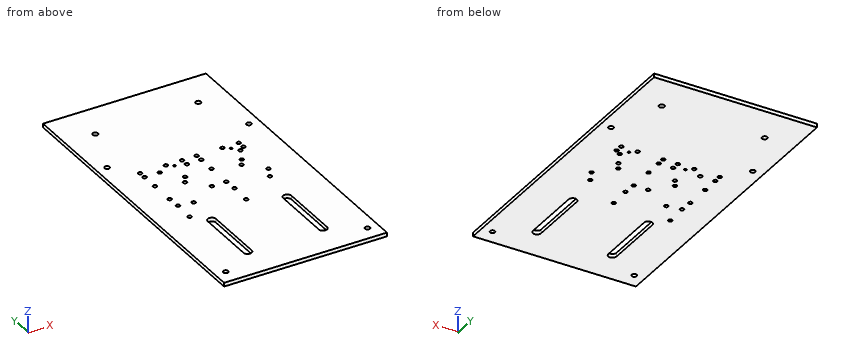
Autodesk Inventor part; units mm, degrees
ref_plane "YZ Plane" through (0, 0, 0) normal (1, 0, 0) x (0, 1, 0)
ref_plane "XZ Plane" through (0, 0, 0) normal (0, 1, 0) x (-1, 0, 0)
ref_plane "XY Plane" through (0, 0, 0) normal (0, 0, 1) x (1, 0, 0)
sketch "Sketch1" plane through (0, 0, 0) normal (0, 0, 1) x (1, 0, 0)
  line L0 (-68.58, -128.7145) -> (68.58, -128.7145)
  line L1 (68.58, -128.7145) -> (68.58, 128.7145)
  line L2 (68.58, 128.7145) -> (-68.58, 128.7145)
  line L3 (-68.58, 128.7145) -> (-68.58, -128.7145)
  line L4 (-68.58, -128.7145) -> (68.58, 128.7145) construction
  line L5 (68.58, -128.7145) -> (-68.58, 128.7145) construction
  point P0 (0, 0)
  dimension "d0" = 137.16
  dimension "d1" = 257.429
extrude "Extrusion1" add sketch "Sketch1" against normal blind 3.175
sketch "Sketch2" plane through (0, 0, 0) normal (0, 0, 1) x (1, 0, 0)
  circle A0 centre (-59.69, 52.5145) radius 2.0955
  line L0 (-68.58, 128.7145) -> (-68.58, -128.7145)
  line L1 (-68.58, 128.7145) -> (68.58, 128.7145)
  circle A1 centre (59.69, 52.5145) radius 2.0955
  line L2 (68.58, -128.7145) -> (68.58, 128.7145)
  circle A2 centre (-59.69, -116.0145) radius 2.0955
  circle A3 centre (59.69, -116.0145) radius 2.0955
  line L3 (-68.58, -128.7145) -> (68.58, -128.7145)
  point P0 (0, 0)
  dimension "d4" = 8.89
  dimension "d5" = 76.2
  dimension "d6" = 76.2
  dimension "d7" = 8.89
  dimension "d8" = 4.191
  dimension "d9" = 12.7
  dimension "d10" = 8.89
  dimension "d11" = 8.89
  dimension "d12" = 12.7
  dimension "d13" = 4.191
  dimension "d21" = 4.191
  dimension "d22" = 4.191
hole "Hole1" at (-59.69, 52.5145, 0) at (59.69, 52.5145, 0) at (-59.69, -116.0145, 0) at (59.69, -116.0145, 0) direction (0, 0, -1) diameter 4.191 end through all
sketch "Sketch4" plane through (0, 0, 0) normal (0, 0, 1) x (1, 0, 0)
  line L0 (-35.179, -49.0855) -> (-35.179, -99.8855)
  line L1 (-28.321, -49.0855) -> (-28.321, -99.8855)
  line L2 (28.321, -49.0855) -> (28.321, -99.8855)
  line L3 (35.179, -49.0855) -> (35.179, -99.8855)
  line L4 (-68.58, 128.7145) -> (-68.58, -128.7145)
  line L5 (68.58, -128.7145) -> (68.58, 128.7145)
  line L6 (-68.58, -128.7145) -> (68.58, -128.7145)
  arc A0 (-28.321, -49.0855) -> (-35.179, -49.0855) centre (-31.75, -49.0855) ccw
  arc A1 (-35.179, -99.8855) -> (-28.321, -99.8855) centre (-31.75, -99.8855) ccw
  arc A2 (35.179, -49.0855) -> (28.321, -49.0855) centre (31.75, -49.0855) ccw
  arc A3 (28.321, -99.8855) -> (35.179, -99.8855) centre (31.75, -99.8855) ccw
  point P0 (0, 0)
  dimension "d23" = 6.858
  dimension "d24" = 6.858
  dimension "d25" = 33.401
  dimension "d26" = 50.8
  dimension "d27" = 33.401
  dimension "d28" = 28.829
  dimension "d29" = 28.829
  dimension "d30" = 28.829
  dimension "d31" = 28.829
  dimension "d32" = 50.8
  dimension "d33" = 50.8
  dimension "d34" = 50.8
extrude "Extrusion2" cut sketch "Sketch4" against normal blind 3.175
sketch "Sketch5" plane through (0, 0, 0) normal (0, 0, 1) x (1, 0, 0)
  line L0 (-68.58, 128.7145) -> (68.58, 128.7145)
  line L1 (68.58, 128.7145) -> (68.58, -128.7145)
  point P0 (0, 0)
  point P1 (-43.3324, 96.9645)
  point P2 (43.3324, 96.9645)
  dimension "d37" = 31.75
  dimension "d38" = 86.6648
  dimension "d39" = 31.75
  dimension "d40" = 25.2476
hole "Hole2" at (-43.3324, 96.9645, 0) at (43.3324, 96.9645, 0) direction (0, 0, -1) diameter 4.4704 end through all
sketch "battery_buzzer" plane through (0, 0, 0) normal (0, 0, 1) x (1, 0, 0)
  line L0 (-50.8, 39.8145) -> (50.8, 39.8145)
  line L1 (50.8, 39.8145) -> (50.8, -36.3855)
  line L2 (50.8, -36.3855) -> (-50.8, -36.3855)
  line L3 (-50.8, -36.3855) -> (-50.8, 39.8145)
  line L4 (68.58, -128.7145) -> (68.58, 128.7145)
  line L5 (68.58, 128.7145) -> (-68.58, 128.7145)
  line L6 (-68.58, 128.7145) -> (-68.58, -128.7145)
  line L7 (-46.99, 37.2745) -> (-13.97, 37.2745)
  line L8 (-13.97, 37.2745) -> (-13.97, 9.3345)
  line L9 (-13.97, 9.3345) -> (-46.99, 9.3345)
  line L10 (-46.99, 9.3345) -> (-46.99, 37.2745)
  circle A0 centre (-43.18, 33.4645) radius 1.651
  circle A1 centre (-43.18, 12.5095) radius 1.651
  circle A2 centre (-17.78, 12.5095) radius 1.651
  line L11 (0.635, 37.2745) -> (33.655, 37.2745)
  line L12 (33.655, 37.2745) -> (33.655, 9.3345)
  line L13 (33.655, 9.3345) -> (0.635, 9.3345)
  line L14 (0.635, 9.3345) -> (0.635, 37.2745)
  circle A3 centre (4.445, 33.4645) radius 1.651
  circle A4 centre (4.445, 12.5095) radius 1.651
  circle A5 centre (29.845, 12.5095) radius 1.651
  point P0 (-1.6153, -4.4833)
  point P1 (48.3688, -4.4833)
  dimension "d48" = 17.78
  dimension "d49" = 88.9
  dimension "d50" = 76.2
  dimension "d51" = 17.78
  dimension "d52" = 33.02
  dimension "d54" = 3.302
  dimension "d55" = 3.302
  dimension "d57" = 3.81
  dimension "d58" = 3.81
  dimension "d59" = 3.81
  dimension "d60" = 20.955
  dimension "d62" = 25.4
  dimension "d74" = 33.02
  dimension "d75" = 3.302
  dimension "d76" = 3.302
  dimension "d77" = 3.81
  dimension "d78" = 3.81
  dimension "d79" = 3.81
  dimension "d80" = 20.955
  dimension "d81" = 25.4
  dimension "d190" = 25.4
  dimension "d191" = 95.25
  dimension "d192" = 73.025
sketch "grizzly_bear" plane through (0, 0, 0) normal (0, 0, 1) x (1, 0, 0)
  line L0 (-5.08, -39.9415) -> (-5.08, 36.2585)
  line L1 (-5.08, 36.2585) -> (-46.355, 36.2585)
  line L2 (-46.355, 36.2585) -> (-46.355, -39.9415)
  line L3 (-46.355, -39.9415) -> (-5.08, -39.9415)
  circle A0 centre (-43.18, -36.8935) radius 1.651
  circle A1 centre (-7.874, 33.4645) radius 1.651
  circle A2 centre (-43.18, 33.4645) radius 1.651
  line L4 (42.545, -39.9415) -> (42.545, 36.2585)
  line L5 (42.545, 36.2585) -> (1.27, 36.2585)
  line L6 (1.27, 36.2585) -> (1.27, -39.9415)
  line L7 (1.27, -39.9415) -> (42.545, -39.9415)
  circle A3 centre (4.445, -36.8935) radius 1.651
  circle A4 centre (39.751, 33.4645) radius 1.651
  circle A5 centre (4.445, 33.4645) radius 1.651
  line L8 (-68.58, 128.7145) -> (-68.58, -128.7145)
  line L9 (68.58, 128.7145) -> (-68.58, 128.7145)
  point P0 (0, 0)
  point P1 (53.9394, 0)
  dimension "d83" = 3.302
  dimension "d85" = 76.2
  dimension "d86" = 41.275
  dimension "d89" = 2.794
  dimension "d90" = 3.175
  dimension "d91" = 2.794
  dimension "d92" = 38.481
  dimension "d97" = 73.152
  dimension "d98" = 3.175
  dimension "d166" = 3.302
  dimension "d168" = 76.2
  dimension "d169" = 41.275
  dimension "d172" = 2.794
  dimension "d173" = 3.175
  dimension "d174" = 2.794
  dimension "d175" = 38.481
  dimension "d180" = 73.152
  dimension "d181" = 3.175
  dimension "d182" = 6.35
  dimension "d188" = 95.25
  dimension "d189" = 25.4
sketch "Smartsensor" plane through (0, 0, 0) normal (0, 0, 1) x (1, 0, 0)
  line L0 (-46.99, 9.3345) -> (-46.99, 37.2745)
  line L1 (-46.99, 37.2745) -> (-13.97, 37.2745)
  line L2 (-13.97, 37.2745) -> (-13.97, 9.3345)
  line L3 (-46.99, 9.3345) -> (-13.97, 9.3345)
  circle A0 centre (-43.18, 33.4645) radius 1.651
  circle A1 centre (-17.78, 12.5095) radius 1.651
  circle A2 centre (-16.51, 29.6545) radius 1
  line L4 (0.635, 9.3345) -> (0.635, 37.2745)
  line L5 (0.635, 37.2745) -> (33.655, 37.2745)
  line L6 (33.655, 37.2745) -> (33.655, 9.3345)
  line L7 (0.635, 9.3345) -> (33.655, 9.3345)
  circle A3 centre (4.445, 33.4645) radius 1.651
  circle A4 centre (29.845, 12.5095) radius 1.651
  circle A5 centre (31.115, 29.6545) radius 1
  point P0 (0, 0)
  point P1 (4.445, 33.4645)
sketch "SmartsensorPowered" plane through (0, 0, 0) normal (0, 0, 1) x (1, 0, 0)
  line L0 (-46.355, 36.6395) -> (-18.415, 36.6395)
  line L1 (-18.415, 36.6395) -> (-18.415, -23.0505)
  line L2 (-18.415, -23.0505) -> (-46.355, -23.0505)
  line L3 (-46.355, -23.0505) -> (-46.355, 36.6395)
  circle A0 centre (-43.18, 33.4645) radius 1.651
  circle A1 centre (-21.59, 33.4645) radius 1.651
  circle A2 centre (-42.545, -19.2405) radius 1.651
  circle A3 centre (-21.59, 6.1595) radius 1.651
  line L4 (-68.58, 128.7145) -> (-68.58, -128.7145)
  line L5 (68.58, 128.7145) -> (-68.58, 128.7145)
  line L6 (1.27, 36.6395) -> (29.21, 36.6395)
  line L7 (29.21, 36.6395) -> (29.21, -23.0505)
  line L8 (29.21, -23.0505) -> (1.27, -23.0505)
  line L9 (1.27, -23.0505) -> (1.27, 36.6395)
  circle A4 centre (4.445, 33.4645) radius 1.651
  circle A5 centre (26.035, 33.4645) radius 1.651
  circle A6 centre (5.08, -19.2405) radius 1.651
  circle A7 centre (26.035, 6.1595) radius 1.651
  dimension "d99" = 59.69
  dimension "d100" = 27.94
  dimension "d101" = 3.302
  dimension "d102" = 3.302
  dimension "d103" = 3.302
  dimension "d104" = 3.302
  dimension "d105" = 3.175
  dimension "d106" = 3.81
  dimension "d107" = 3.175
  dimension "d108" = 3.81
  dimension "d109" = 3.175
  dimension "d110" = 3.175
  dimension "d111" = 3.175
  dimension "d112" = 30.48
  dimension "d186" = 25.4
  dimension "d187" = 95.25
  dimension "d193" = 59.69
  dimension "d194" = 27.94
  dimension "d195" = 3.302
  dimension "d196" = 3.302
  dimension "d197" = 3.302
  dimension "d198" = 3.302
  dimension "d199" = 3.175
  dimension "d200" = 3.81
  dimension "d201" = 3.175
  dimension "d202" = 3.81
  dimension "d203" = 3.175
  dimension "d204" = 3.175
  dimension "d205" = 3.175
  dimension "d206" = 30.48
  dimension "d207" = 73.025
sketch "teamflag" plane through (0, 0, 0) normal (0, 0, 1) x (1, 0, 0)
  line L0 (-45.72, 29.6545) -> (-5.08, 29.6545)
  line L1 (-5.08, 29.6545) -> (-5.08, -10.9855)
  line L2 (-5.08, -10.9855) -> (-45.72, -10.9855)
  line L3 (-45.72, -10.9855) -> (-45.72, 29.6545)
  circle A0 centre (-43.18, 27.1145) radius 1.651
  circle A1 centre (-43.18, -8.4455) radius 1.651
  circle A2 centre (-7.62, 27.1145) radius 1.651
  circle A3 centre (-7.62, -8.4455) radius 1.651
  line L4 (1.905, 29.6545) -> (42.545, 29.6545)
  line L5 (42.545, 29.6545) -> (42.545, -10.9855)
  line L6 (42.545, -10.9855) -> (1.905, -10.9855)
  line L7 (1.905, -10.9855) -> (1.905, 29.6545)
  circle A4 centre (4.445, 27.1145) radius 1.651
  circle A5 centre (4.445, -8.4455) radius 1.651
  circle A6 centre (40.005, 27.1145) radius 1.651
  circle A7 centre (40.005, -8.4455) radius 1.651
  line L8 (-68.58, 128.7145) -> (-68.58, -128.7145)
  line L9 (68.58, 128.7145) -> (-68.58, 128.7145)
  point P0 (0, 0)
  point P1 (-43.18, 33.4645)
  point P2 (4.445, 33.4645)
  point P3 (-42.545, -19.2405)
  point P4 (5.08, -19.2405)
  point P5 (-43.18, 33.4645)
  point P6 (4.445, 27.1145)
  dimension "d128" = 40.64
  dimension "d129" = 40.64
  dimension "d140" = 35.56
  dimension "d141" = 35.56
  dimension "d142" = 35.56
  dimension "d143" = 2.54
  dimension "d144" = 2.54
  dimension "d145" = 40.64
  dimension "d146" = 40.64
  dimension "d147" = 35.56
  dimension "d148" = 35.56
  dimension "d149" = 35.56
  dimension "d150" = 2.54
  dimension "d151" = 2.54
  dimension "d209" = 25.4
  dimension "d210" = 101.6
  dimension "d211" = 73.025
  dimension "d212" = 101.6
sketch "cape" plane through (0, 0, 0) normal (0, 0, 1) x (1, 0, 0)
  line L0 (-33.655, 30.2793) -> (38.4048, 30.2793)
  line L1 (38.4048, 30.2793) -> (38.4048, -24.3205)
  line L2 (38.4048, -24.3205) -> (-33.655, -24.3205)
  line L3 (-33.655, -24.3205) -> (-33.655, 30.2793)
  circle A0 centre (-30.48, 27.1145) radius 1.5875
  circle A1 centre (-30.48, -21.1455) radius 1.5875
  circle A2 centre (35.56, 23.9395) radius 1.5875
  circle A3 centre (35.56, -17.9705) radius 1.5875
  line L4 (-68.58, 128.7145) -> (-68.58, -128.7145)
  point P0 (0, 0)
  point P1 (-43.18, 33.4645)
  point P2 (-43.18, 27.1145)
  point P3 (-42.545, -19.2405)
  point P4 (-30.48, 27.1145)
  point P5 (-24.13, 20.7645)
  dimension "d152" = 3.175
  dimension "d153" = 72.0598
  dimension "d154" = 54.5998
  dimension "d155" = 48.26
  dimension "d156" = 0
  dimension "d157" = 3.175
  dimension "d158" = 3.175
  dimension "d159" = 41.91
  dimension "d160" = 0
  dimension "d161" = 6.35
  dimension "d162" = 2.8448
  dimension "d269" = 38.1
  dimension "d270" = 44.45
sketch "Board Area" plane through (0, 0, 0) normal (0, 0, 1) x (1, 0, 0)
  line L0 (-50.8, 39.8145) -> (50.8, 39.8145)
  line L1 (50.8, 39.8145) -> (50.8, -128.7145)
  line L2 (50.8, -128.7145) -> (-50.8, -128.7145)
  line L3 (-50.8, -128.7145) -> (-50.8, 39.8145)
  line L4 (68.58, 128.7145) -> (-68.58, 128.7145)
  line L5 (-68.58, 128.7145) -> (-68.58, -128.7145)
  line L6 (-68.58, -128.7145) -> (68.58, -128.7145)
  point P0 (0, 0)
  dimension "d163" = 101.6
  dimension "d164" = 88.9
  dimension "d165" = 17.78
hole "Hole3" at (-43.18, 27.1145, 0) at (-43.18, -8.4455, 0) at (-7.62, -8.4455, 0) at (-7.62, 27.1145, 0) at (4.445, 27.1145, 0) at (4.445, -8.4455, 0) at (40.005, -8.4455, 0) at (40.005, 27.1145, 0) direction (0, 0, -1) diameter 3.302 end through all
hole "Hole5" at (-43.18, -36.8935, 0) at (4.445, -36.8935, 0) at (39.751, 33.4645, 0) at (-7.874, 33.4645, 0) direction (0, 0, -1) diameter 3.302 end through all
hole "Hole6" at (-17.78, 12.5095, 0) at (29.845, 12.5095, 0) direction (0, 0, -1) diameter 3.302 end through all
hole "Hole7" at (-43.18, 12.5095, 0) at (4.445, 12.5095, 0) direction (0, 0, -1) diameter 3.302 end through all
hole "Hole9" at (-43.18, 33.4645, 0) at (4.445, 33.4645, 0) at (-16.51, 29.6545, 0) direction (0, 0, -1) diameter 2.0066 end through all
hole "Hole10" at (31.115, 29.6545, 0) direction (0, 0, -1) diameter 2.0066 end through all
hole "Hole11" at (-30.48, 27.1145, 0) at (-30.48, -21.1455, 0) at (35.56, -17.9705, 0) at (35.56, 23.9395, 0) direction (0, 0, -1) diameter 3.302 end through all
hole "Hole12" at (-42.545, -19.2405, 0) at (-21.59, 33.4645, 0) at (26.035, 33.4645, 0) at (5.08, -19.2405, 0) at (4.445, 33.4645, 0) at (-43.18, 33.4645, 0) at (-21.59, 6.1595, 0) at (26.035, 6.1595, 0) direction (0, 0, -1) diameter 3.302 end through all
Geometry: final body of the model. Coordinates: model frame, mm. Coordinates: 2 decimals unless noted, no trailing zeros. Loops run counter-clockwise (first coordinate to the right, second up) from the corner with the lowest first, then second, coordinate; pieces in that order, holes last. Notation, with made-up numbers: M 27.25,71.25 L 60.25,71.25 A33 ccw 60.25,110.25 Z; hole C -32,-25 d6. An arc over 180 degrees is marked long. One line per item, written item: value. Start each with the question number.
1) Cut plane B-B (z = -2.25). Count the separate pieces of the cut face and the enclosed holes in it, then the cut area to 3 significant figures.
2) Cut plane A-A (y = -73). Return loops of the section in (x, z) (3 decimals).
3) Pin query (flat end, axial travel): P1, Ø2.5, axis at x = 4.44, y = 33.46, coming from the -Z side. Return the tip coordinate at first contact, or that it passes through.
4) Material intervals for L1, parallel to X at y = 6, z = -2.9; L2, parallel to X at y = -65.5, z = -0.4; L3, parallel to Y at x = -60, z = -3, sorted ascending. Write a range as from..to.
Evaluation:
1. separate pieces: 1
1. enclosed holes: 38
1. area: 34,200 mm^2
2. outline: M -68.58,-3.175 L -35.179,-3.175 L -35.179,0 L -68.58,0 Z; M -28.321,-3.175 L 28.321,-3.175 L 28.321,0 L -28.321,0 Z; M 35.179,-3.175 L 68.58,-3.175 L 68.58,0 L 35.179,0 Z
3. P1: through
4. L1: -68.58..-23.23, -19.95..24.39, 27.68..68.58
4. L2: -68.58..-35.18, -28.32..28.32, 35.18..68.58
4. L3: -128.71..-118.09, -113.94..50.44, 54.59..128.71
